```python
from build123d import *

# Parameters (mm, degrees)
SKETCH1_R           = 1.5875
BOSS_EXTRUDE1_DEPTH = 3.175


with BuildPart() as part:
    # Sketch1 → Boss-Extrude1 (new body)
    with BuildSketch(Plane(origin=(0, 0, 0), x_dir=(1, 0, 0), z_dir=(0, 1, 0))):
        with BuildLine():
            Line((3.175, 0), (123.825, 0))
            ThreePointArc((123.825, 0), (126.07006403, 0.92993597), (127, 3.175))
            Line((127, 3.175), (127, 98.425))
            ThreePointArc((127, 98.425), (126.07006403, 100.67006403), (123.825, 101.6))
            Line((123.825, 101.6), (3.175, 101.6))
            ThreePointArc((3.175, 101.6), (0.92993597, 100.67006403), (0, 98.425))
            Line((0, 98.425), (0, 3.175))
            ThreePointArc((0, 3.175), (0.92993597, 0.92993597), (3.175, 0))
        make_face()
        with Locations((12.7, 54.229148011)):
            Circle(SKETCH1_R, mode=Mode.SUBTRACT)
        with Locations((5.08, 96.52)):
            Circle(SKETCH1_R, mode=Mode.SUBTRACT)
        with Locations((5.08, 5.08)):
            Circle(SKETCH1_R, mode=Mode.SUBTRACT)
        with Locations((121.92, 96.52)):
            Circle(SKETCH1_R, mode=Mode.SUBTRACT)
        with Locations((121.92, 5.08)):
            Circle(SKETCH1_R, mode=Mode.SUBTRACT)
        with BuildLine():
            Line((63.5, 81.216648011), (114.3, 81.216648011))
            ThreePointArc((114.3, 81.216648011), (115.8875, 79.629148011), (114.3, 78.041648011))
            Line((114.3, 78.041648011), (63.5, 78.041648011))
            ThreePointArc((63.5, 78.041648011), (61.9125, 79.629148011), (63.5, 81.216648011))
        make_face(mode=Mode.SUBTRACT)
        with BuildLine():
            Line((63.5, 55.816648011), (114.3, 55.816648011))
            ThreePointArc((114.3, 55.816648011), (115.8875, 54.229148011), (114.3, 52.641648011))
            Line((114.3, 52.641648011), (63.5, 52.641648011))
            ThreePointArc((63.5, 52.641648011), (61.9125, 54.229148011), (63.5, 55.816648011))
        make_face(mode=Mode.SUBTRACT)
        with BuildLine():
            ThreePointArc((12.7, 78.041648011), (36.5125, 54.229148011), (12.7, 30.416648011))
            ThreePointArc((12.7, 30.416648011), (11.1125, 28.829148011), (12.7, 27.241648011))
            ThreePointArc((12.7, 27.241648011), (39.6875, 54.229148011), (12.7, 81.216648011))
            ThreePointArc((12.7, 81.216648011), (11.1125, 79.629148011), (12.7, 78.041648011))
        make_face(mode=Mode.SUBTRACT)
    extrude(amount=BOSS_EXTRUDE1_DEPTH)


solid = part.part
```
Work out the finished part from the listing and answer in its coordinate system (mm). A direction names the side the tool comes from. Coordinates: 2 decimals unless noted, no trailing zeros. Loops run counter-clockwise (first coordinate to the right, second up) from the corner with the lowest first, then second, coordinate; pieces in that order, holes last. Notation, with made-up numbers: (71, 8) - (97, 8) arc R22 ccw to (97, 25) - close; hole circle Ø1 at (86.5, -39). An arc over 180 degrees is marked (long way). Use a Markdown table: item, result.
Item 1: For faces 4 (the cylindrical face through (61.913, 1.565, -54.194)), 5 (the flat face through (127, 2, -50)), determine the directions among +Z, -Z, +X, -X, +Y, -Y from which every point of the face is accessible in a straight line to the end or side of a thin tool.
Evaluation:
| item | result |
|---|---|
| face 4 | +Y, -Y |
| face 5 | +Z, -Z, +X, +Y, -Y |
Item 2: Find section B-B, the plane x = 5.08. Determine the outline of the cut face in (y, z) (1 decimal).
Evaluation:
| item | result |
|---|---|
| outline | (0, -101.6) - (3.2, -101.6) - (3.2, -98.1) - (0, -98.1) - close; (0, -94.9) - (3.2, -94.9) - (3.2, -6.7) - (0, -6.7) - close; (0, -3.5) - (3.2, -3.5) - (3.2, 0) - (0, 0) - close |
Item 3: Find section A-A, the plane z = -96.52. Determine the outline of the cut face in (x, y) (1 decimal), and give its area (3 significant figures).
Evaluation:
| item | result |
|---|---|
| outline | (0, 0) - (3.5, 0) - (3.5, 3.2) - (0, 3.2) - close; (6.7, 0) - (120.3, 0) - (120.3, 3.2) - (6.7, 3.2) - close; (123.5, 0) - (127, 0) - (127, 3.2) - (123.5, 3.2) - close |
| area | 383 mm2 |
Item 4: Consider probe 1 along Z at (x, y) = (121.92, 1.1); probe 2 along X at (y, z) = (1.85, -5.08); probe 3 along Z at (x, y) = (88, 2.15). Determine where each line is inside the solid, lowest interval first. Write a range as from..to.
Evaluation:
| item | result |
|---|---|
| probe 1 | z = -101.6..-98.11, -94.93..-6.67, -3.49..0 |
| probe 2 | x = 0..3.49, 6.67..120.33, 123.51..127 |
| probe 3 | z = -101.6..-81.22, -78.04..-55.82, -52.64..0 |
Item 5: Find section C-C, the plane y = 1.2. State how many separate pieces and enclosed holes the cut face has, and give its area (3 significant figures).
Evaluation:
| item | result |
|---|---|
| separate pieces | 1 |
| enclosed holes | 8 |
| area | 12,300 mm2 |
Item 6: The mould has two halves that part along Z. Classify faces 1 (the flat face through (63, 0, -52)), 2 (the cylindrical face through (0.95, 1.57, -100.69)), 3 (the cylindrical face through (6.594, 1.565, -5.557)): +Z half, -Z half, draft (parallel to the pull), parting line (faces both ways), or undercut.
Evaluation:
| item | result |
|---|---|
| face 1 | draft |
| face 2 | -Z half |
| face 3 | undercut |
